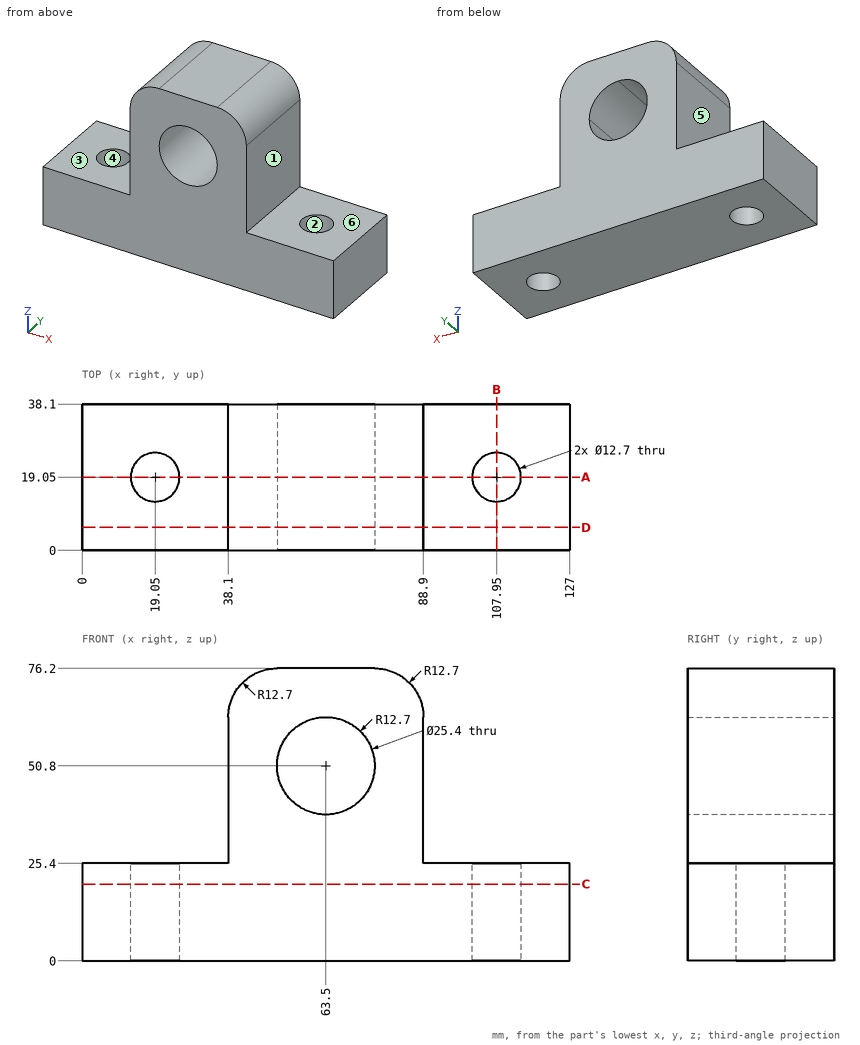
Check sheet for the drawn part. Datum: minimum x, y, z corner. Units: mm. A direction names the side the tool comes from. Coordinates: 2 decimals unless noted, no trailing zeros. Order: outer loops, then holes, each group sorted by start corner. A loop starts at its lowest first (then second) coordinate and runs counter-clockwise, first axis right, second up. Notation, with made-up numbers: (29.5, -32.75) -> (80.5, -32.75) arc R29 ccw to (80.5, -11.75) -> close; hole circle Ø10 at (-6.5, 42). An arc over 180 degrees is marked (long way). Use a Markdown table: item, result. Add a question column.
1. Cross-section at A-A (y = 19.05). Enter the section's corners in (x, z), and give its area (3 significant figures).
2. Cross-section at D-D (y = 6). Enter the section's corners in (x, z), and give its area (3 significant figures).
3. Go/stop test with flat-tipped pins: pin 1 Ø6 at (y, z) = (7, 34.5) entering from +X; pin 2 Ø19 at (y, z) = (10.5, 48.5) entering from -X; pin 3 Ø19 at (x, y) = (10, 27.5) entering from +Z. Record where each tip stops, or that it passes through.
4. Cross-section at C-C (z = 20). Enter the section's corners in (x, y), and give its area (3 significant figures).
5. Mould release check, pull along X, two halves, no side actions. Record for the marked faces 4, 5 and 6: pulls with the +X half, pulls with the -X half, needs draft (parallel to the pull), parting line crosses it, or undercut.
6. Set-up check for the marked faces 1, 2 and 3: record each of +Z, -Z, +X, -X, +Y, -Y from which the full face is reachable in a straight line by a thin tool's end or side.
7. Material ranges on L1, parallel to X at y = 19, z = 15; L2, parallel to Y at x = 107.95, z = 14.25; L3, parallel to X at y = 13.5, z = 23.5, recorded low to high.
8. Cross-section at B-B (x = 107.95). Enter the section's corners in (y, z), and give its area (3 significant figures).
Filled sheet:
| question | item | result |
|---|---|---|
| 1 | outline | (0, 0) -> (12.7, 0) -> (12.7, 25.4) -> (0, 25.4) -> close; (25.4, 0) -> (101.6, 0) -> (101.6, 25.4) -> (88.9, 25.4) -> (88.9, 63.5) arc R12.7 ccw to (76.2, 76.2) -> (50.8, 76.2) arc R12.7 ccw to (38.1, 63.5) -> (38.1, 25.4) -> (25.4, 25.4) -> close; (114.3, 0) -> (127, 0) -> (127, 25.4) -> (114.3, 25.4) -> close; hole circle Ø25.4 at (63.5, 50.8) |
| 1 | area | 4,590 mm2 |
| 2 | outline | (0, 0) -> (127, 0) -> (127, 25.4) -> (88.9, 25.4) -> (88.9, 63.5) arc R12.7 ccw to (76.2, 76.2) -> (50.8, 76.2) arc R12.7 ccw to (38.1, 63.5) -> (38.1, 25.4) -> (0, 25.4) -> close; hole circle Ø25.4 at (63.5, 50.8) |
| 2 | area | 5,230 mm2 |
| 3 | pin 1 | x = 88.9 |
| 3 | pin 2 | x = 38.1 |
| 3 | pin 3 | z = 25.4 |
| 4 | outline | (0, 0) -> (127, 0) -> (127, 38.1) -> (0, 38.1) -> close; hole circle Ø12.7 at (19.05, 19.05); hole circle Ø12.7 at (107.95, 19.05) |
| 4 | area | 4,590 mm2 |
| 5 | face 4 | undercut |
| 5 | face 5 | pulls with the -X half |
| 5 | face 6 | needs draft |
| 6 | face 1 | +Z, +X, +Y, -Y |
| 6 | face 2 | +Z, -Z |
| 6 | face 3 | +Z, -X, +Y, -Y |
| 7 | L1 | 0 to 12.7, 25.4 to 101.6, 114.3 to 127 |
| 7 | L2 | 0 to 12.7, 25.4 to 38.1 |
| 7 | L3 | 0 to 15.96, 22.14 to 104.86, 111.04 to 127 |
| 8 | outline | (0, 0) -> (12.7, 0) -> (12.7, 25.4) -> (0, 25.4) -> close; (25.4, 0) -> (38.1, 0) -> (38.1, 25.4) -> (25.4, 25.4) -> close |
| 8 | area | 645 mm2 |
